from build123d import *

# Parameters (mm, degrees)
F2_R = 1


# Not quite as in the source:
# - two fillets or chamfers of one size are made in one step


with BuildPart() as f1:
    # F0 (on Front) → F1 (revolve)
    with BuildSketch(Plane.XZ):
        Polygon((-10.4996741857, -0.0827163458), (0, 0), (0, 69.9172836542), (0, 70.5213546753), (-6.2381645857, 70.5213546753), (-6.5643620988, 69.9172836542), (-7.2255664847, 69.2085400224), (-8.7180831586, 69.2085400224), (-9.2690859436, 69.9172836542), (-10.4996741857, 69.9172836542), align=None)
    revolve(axis=Axis((0, 0, 34.9586418271), (0, 0, 1)))

    # F2
    f2_edges = [f1.edges().sort_by_distance(p)[0] for p in [
        (10.499674, 0, -0.082716),
        (6.238165, 0, 70.521355),
        (10.499674, 0, 69.917284),
    ]]
    fillet(f2_edges, radius=F2_R)


solid = f1.part
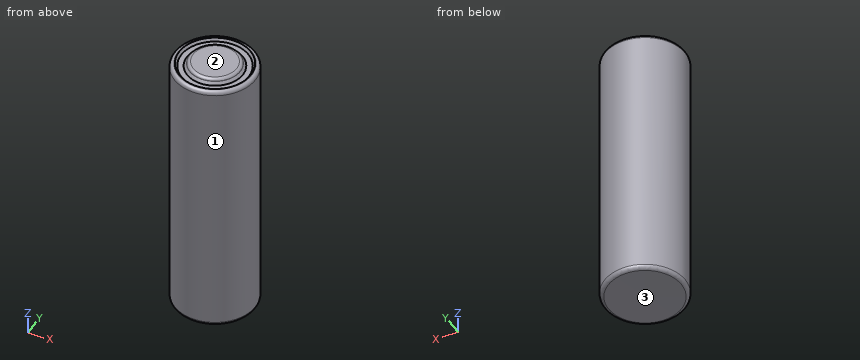
Input: part model. Units: mm. Frame: model coordinates. Face numbers are marked on the shaded views. Coordinates: 2 decimals unless noted, no trailing zeros. Order: outer loops, then holes, each group sorted by start corner. A loop starts at its lowest first (then second) coordinate and runs counter-clockwise, first axis right, second up. Notation, with made-up numbers: M 35.25,32 L 75.25,32 A16 cw 75.25,39 Z; hole C -24.75,-32.75 d8. An arc over 180 degrees is marked long. Write item = value, one per line. Start each with the question number.
(1) Pull-direction query (Y, two-part tool) for the marked faces 1, 2 and 3; classes: released by +Y, released by -Y, zero draft, split by the parting line, or undercut.
(2) Line query: line 1 along Z through (x, y) = (9, -2.25); line 2 along Z through (x, y) = (1.5, 7.5); line 3 along Y through (x, z) = (-4.5, 13). Output: solid intervals per line, ascending. Write a range as [from, to].
(3) Section A-A on z = 27. Output: boundary loops of the cut face in (x, y).
(4) First-contact query: P1, Ø8, axis at x = -5, z = 50, coming from the -Y side; P2, Ø2, axis at y = -2.5, z = 8.5, coming from the +X side; P3, Ø1, axis at y = 7.5, z = 24, coming from the -X side. Flat tips, straight axial feed; report the tip coordinate or a pass-through.
Result set:
q1.face_1 = split by the parting line
q1.face_2 = zero draft
q1.face_3 = undercut
q2.line_1 = [-0.07, 69.92]
q2.line_2 = [-0.06, 69.21]
q2.line_3 = [-9.49, 9.49]
q3.outline = C 0,0 d21
q4.P1 = -10.45
q4.P2 = 10.39
q4.P3 = -7.83
